```python
from build123d import *

# Parameters (mm, degrees)
BOSS_EXTRUDE1_DEPTH = 5.5
SKETCH3_R           = 1.5875
CUT_EXTRUDE1_DEPTH  = 9.525


with BuildPart() as part:
    # Sketch1 → Boss-Extrude1 (new body)
    with BuildSketch(Plane.XY):
        Polygon((0, 0), (-3, 0), (-3, 15), (0, 15), (0, 9), (3.525, 9), (3.525, 15), (6.525, 15), (6.525, 0), (3.525, 0), (3.525, 6), (0, 6), align=None)
    extrude(amount=BOSS_EXTRUDE1_DEPTH)

    # Sketch3 → Cut-Extrude1 (cut)
    with BuildSketch(Plane.ZY.offset(3)):
        with BuildLine():
            Line((5.5, 15), (2.75, 15))
            ThreePointArc((2.75, 15), (4.694543648, 14.194543648), (5.5, 12.25))
            Line((5.5, 12.25), (5.5, 15))
        make_face()
        with BuildLine():
            Line((0, 15), (0, 12.25))
            ThreePointArc((0, 12.25), (0.805456352, 14.194543648), (2.75, 15))
            Line((2.75, 15), (0, 15))
        make_face()
        with Locations((2.75, 12)):
            Circle(SKETCH3_R)
        with Locations((2.75, 3)):
            Circle(SKETCH3_R)
        with BuildLine():
            ThreePointArc((2.75, 0), (0.805456352, 0.805456352), (0, 2.75))
            Line((0, 2.75), (0, 0))
            Line((0, 0), (2.75, 0))
        make_face()
        with BuildLine():
            ThreePointArc((2.75, 0), (4.694543648, 0.805456352), (5.5, 2.75))
            Line((5.5, 2.75), (5.5, 0))
            Line((5.5, 0), (2.75, 0))
        make_face()
    extrude(amount=-CUT_EXTRUDE1_DEPTH, mode=Mode.SUBTRACT)


solid = part.part
```
Part model, mm, in its own coordinate system. A direction names the side the tool comes from. Give positions to 0.01 mm unless a question says otherwise; leave off trailing zeros. Order: outer loops, then holes, each group sorted by start corner. A loop starts at its lowest first (then second) coordinate and runs counter-clockwise, first axis right, second up. Notation, with made-up numbers: M 89.25,52 L 116.25,52 A24 cw 116.25,71 Z; hole C -22.5,31.5 d5. An arc over 180 degrees is marked long. Use a Markdown table: item, result. Add a question column.
(1) Drop a flat-ended pin along its axis: P1, Ø3, axis at y = 12, z = 2.75, coming from the +X side. Give the stop position or say it passes through.
(2) Saw through at B-B, the plane x = 5.5. Give the number of separate pieces and of enclosed holes in the cut face, and give its area (3 significant figures).
(3) Saw through at D-D, the plane y = 3.25. Give the cut face in (x, z) (3 decimals), and give its area (3 significant figures).
(4) Saw through at A-A, the plane y = 12. Give the cut face in (x, z) (1 decimal).
(5) 3-axis set-ups, long thin cutter, end or side, ignore diameter. For faces 1 (the face through (0, 10.71, 3.93)), 2 (the face through (3.525, 4.29, 3.93)), 3 (the face through (-1.52, 10.45, 2.41)): which of +Z, -Z, +X, -X, +Y, -Y reach the whole face in a straight line?
(6) Probe line 1 along Y through (x, z) = (-0.9, 2.75); line 2 along X through (y, z) = (5.5, 2.1) (3 decimals); line 3 along Y through (x, z) = (-2.25, 2.1). List the from-to ranges inside material, lowest first. Write a range as [from, to].
(7) Mould opens along Z. For faces 4 (the face through (-1.521, 2.034, 1.49)), 5 (the face through (2, 8, 5.5)), 6 (the face through (5.004, 2.034, 1.49)), 7 (the face through (0, 4.4, 3.9)) say: +Z half, -Z half, draft (parallel to the pull), parting line (faces both ways), or undercut.
(8) Saw through at C-C, the plane z = 1.65. Give the cut face in (x, y) (3 decimals), and give its area (3 significant figures).
Answer key:
| question | item | result |
|---|---|---|
| 1 | P1 | through |
| 2 | separate pieces | 1 |
| 2 | enclosed holes | 2 |
| 2 | area | 60.2 mm^2 |
| 3 | outline | M -3,0 L 0,0 L 0,1.182 L -3,1.182 Z; M -3,4.318 L 0,4.318 L 0,5.5 L -3,5.5 Z; M 3.525,0 L 6.525,0 L 6.525,1.182 L 3.525,1.182 Z; M 3.525,4.318 L 6.525,4.318 L 6.525,5.5 L 3.525,5.5 Z |
| 3 | area | 14.2 mm^2 |
| 4 | outline | M -3,0 L 0,0 L 0,1.2 L -3,1.2 Z; M -3,4.3 L 0,4.3 L 0,5.5 L -3,5.5 Z; M 3.5,0 L 6.5,0 L 6.5,1.2 L 3.5,1.2 Z; M 3.5,4.3 L 6.5,4.3 L 6.5,5.5 L 3.5,5.5 Z |
| 5 | face 1 | +Z, -Z, +Y |
| 5 | face 2 | +Z, -Z, -Y |
| 5 | face 3 | +X, -X |
| 6 | line 1 | [0, 1.41], [4.59, 10.41], [13.59, 15] |
| 6 | line 2 | [-3, 0], [3.525, 6.525] |
| 6 | line 3 | [0.08, 1.55], [4.45, 10.55], [13.45, 14.92] |
| 7 | face 4 | undercut |
| 7 | face 5 | +Z half |
| 7 | face 6 | undercut |
| 7 | face 7 | draft |
| 8 | outline | M -3,0.23 L 0,0.23 L 0,1.855 L -3,1.855 Z; M -3,4.145 L 0,4.145 L 0,6 L 3.525,6 L 3.525,4.145 L 6.525,4.145 L 6.525,10.855 L 3.525,10.855 L 3.525,9 L 0,9 L 0,10.855 L -3,10.855 Z; M -3,13.145 L 0,13.145 L 0,14.77 L -3,14.77 Z; M 3.525,0.23 L 6.525,0.23 L 6.525,1.855 L 3.525,1.855 Z; M 3.525,13.145 L 6.525,13.145 L 6.525,14.77 L 3.525,14.77 Z |
| 8 | area | 70.3 mm^2 |
